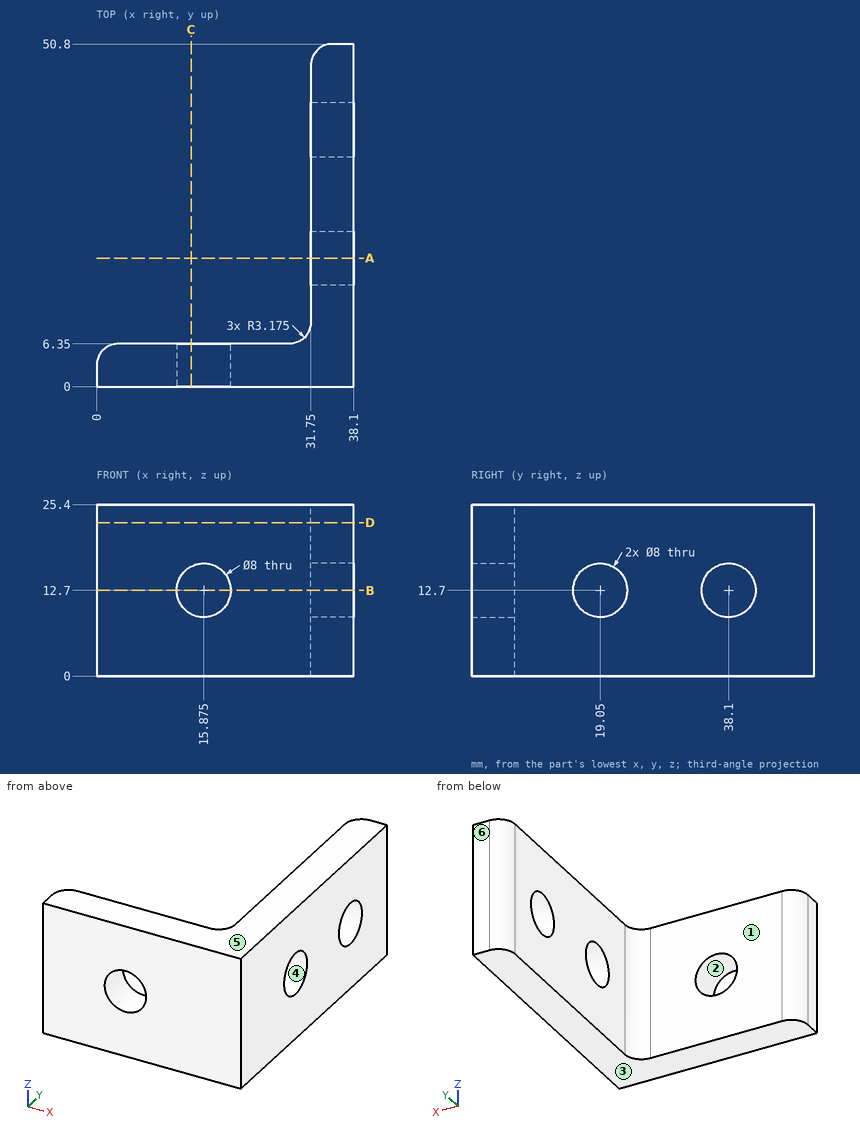
Job drawing, mm, ordinate dimensions from the low corner. One solid piece. A direction names the side the tool comes from. Coordinates: 2 decimals unless noted, no trailing zeros. Order: outer loops, then holes, each group sorted by start corner. A loop starts at its lowest first (then second) coordinate and runs counter-clockwise, first axis right, second up. Notation, with made-up numbers: (59.25, 73.5) - (102.25, 73.5) arc R22 ccw to (102.25, 102.5) - close; hole circle Ø7 at (3, 36.5). An arc over 180 degrees is marked (long way). Return JSON: item names as keys, results as strings. Group by question number.
1) Saw through at D-D, the plane z = 22.75. Write the cut outline in (x, y) (3 decimals).
2) Mould opens along Z. For the marked faces 3, 4, 5 and 6 say: released by +Z, released by -Z, zero draft, split by the parting line, or undercut.
3) Probe line 1 (Z direction, x = 33.75, y = 19.05); line 2 (Y direction, x = 34, z = 9.75); line 3 (Y direction, x = 27, z = 20.5). List the from-to ranges inside material, lowest first. Write a range as from..to.
4) Tool access for the marked faces 1 and 2: list every direction of +Z, -Z, +X, -X, +Y, -Y with a clear straight run to the whole face (end or side of a thin tool).
5) Saw through at B-B, the plane z = 12.7. Write the cut outline in (x, y) (3 decimals).
6) Flat gauge pins, fed straight in: P1, Ø9, axis at y = 38.1, z = 12.7, coming from the -X side; P2, Ø3, axis at x = 22.5, z = 5.5, coming from the +Y side. Where does each tip first touch, or does it go through?
7) Saw through at A-A, the plane y = 19.05. Write the cut outline in (x, z).
8) Saw through at C-C, the plane x = 14. Write the cut outline in (y, z).
Values found:
{
 "1": {"outline": "(0, 0) - (38.1, 0) - (38.1, 50.8) - (34.925, 50.8) arc R3.175 ccw to (31.75, 47.625) - (31.75, 9.525) arc R3.175 cw to (28.575, 6.35) - (3.175, 6.35) arc R3.175 ccw to (0, 3.175) - close"},
 "2": {"face 3": "released by -Z", "face 4": "undercut", "face 5": "released by +Z", "face 6": "zero draft"},
 "3": {"line 1": "z = 0..8.7, 16.7..25.4", "line 2": "y = 0..16.35, 21.75..35.4, 40.8..50.66", "line 3": "y = 0..6.35"},
 "4": {"face 1": "+Z, -Z, -X, +Y", "face 2": "+Y, -Y"},
 "5": {"outline": "(0, 0) - (11.875, 0) - (11.875, 6.35) - (3.175, 6.35) arc R3.175 ccw to (0, 3.175) - close; (19.875, 0) - (38.1, 0) - (38.1, 15.05) - (31.75, 15.05) - (31.75, 9.525) arc R3.175 cw to (28.575, 6.35) - (19.875, 6.35) - close; (31.75, 23.05) - (38.1, 23.05) - (38.1, 34.1) - (31.75, 34.1) - close; (31.75, 42.1) - (38.1, 42.1) - (38.1, 50.8) - (34.925, 50.8) arc R3.175 ccw to (31.75, 47.625) - close"},
 "6": {"P1": "stops at x = 31.75", "P2": "stops at y = 6.35"},
 "7": {"outline": "(31.75, 0) - (38.1, 0) - (38.1, 8.7) - (31.75, 8.7) - close; (31.75, 16.7) - (38.1, 16.7) - (38.1, 25.4) - (31.75, 25.4) - close"},
 "8": {"outline": "(0, 0) - (6.35, 0) - (6.35, 9.17) - (0, 9.17) - close; (0, 16.23) - (6.35, 16.23) - (6.35, 25.4) - (0, 25.4) - close"}
}
